Verification items for the finished model (mm, model axes). Coordinates: 2 decimals unless noted, no trailing zeros. Order: outer loops, then holes, each group sorted by start corner. A loop starts at its lowest first (then second) coordinate and runs counter-clockwise, first axis right, second up. Notation, with made-up numbers: (49.25, 26.5) -> (78.25, 26.5) arc R20 cw to (78.25, 44.5) -> close; hole circle Ø8 at (62, 29). An arc over 180 degrees is marked (long way). Write item = value, one per line. Start each with the question number.
1. Release check for a two-part mould opening along Z. For faces 1 (the cylindrical face through (0, 2, -1)), 2 (the cylindrical face through (0.108, -0.056, 0.488)), 3 (the flat face through (-1, 0, -1)) record: +Z half, -Z half, draft (parallel to the pull), parting line (faces both ways), or undercut.
2. Cross-section at A-A on x = 0. Record the cut outline in (y, z), plus the area to 3 significant figures.
3. Cross-section at B-B on y = -3. Record the cut outline in (x, z), plus the area to 3 significant figures.
4. Thickness scan on line 1 along Z through (x, y) = (0, 1); line 2 along Z through (x, y) = (-0.3, -2.75). Record the ranges inside material, lowest first. Write a range as from..to.
5. Go/stop test with flat-tipped pins: P1, Ø1, axis at y = 0, z = 1, coming from the -X side; P2, Ø1.5, axis at x = 1.5, y = -2.5, coming from the -Z side. Record where each tip stops, or that it passes through.
6. Cross-section at C-C on y = 1.25. Record the cut outline in (x, z), plus the area to 3 significant figures.
Autodesk Inventor part; units mm, degrees
ref_plane "工作平面1" through (0, -4, 0) normal (0, 1, 0) x (-1, 0, 0)
ref_plane "YZ Plane" through (0, 0, 0) normal (1, 0, 0) x (0, 1, 0)
ref_plane "XY Plane" through (0, 0, 0) normal (0, 0, 1) x (1, 0, 0)
sketch "草图1" plane through (0, 0, 0) normal (0, 1, 0) x (-1, 0, 0)
  circle A0 centre (0, 0) radius 2
  dimension "d0" = 4
ref_plane "工作平面1" through (0, -4, 0) normal (0, 1, 0) x (-1, 0, 0)
sketch "草图2" plane through (0, -4, 0) normal (0, 1, 0) x (-1, 0, 0)
  circle A0 centre (0, 0) radius 1
  dimension "d2" = 2
loft "放样1" add profiles "草图1", "草图2"
sketch "草图3" plane through (0, 0, 0) normal (0, 1, 0) x (1, 0, 0)
  circle A0 centre (0, 0) radius 1
  dimension "d7" = 2
extrude "拉伸1" add sketch "草图3" along normal blind 4
sketch "草图4" plane through (0, -4, 0) normal (0, 1, 0) x (-1, 0, 0)
  circle A0 centre (0, 0) radius 0.5
  dimension "d10" = 1
extrude "拉伸2" cut sketch "草图4" along normal through all
properties part number "conver"
Worked out:
q1.face_1 = parting line
q1.face_2 = undercut
q1.face_3 = draft
q2.outline = (-4, -1) -> (0, -2) -> (0, -1) -> (4, -1) -> (4, -0.5) -> (-4, -0.5) -> close; (-4, 0.5) -> (4, 0.5) -> (4, 1) -> (0, 1) -> (0, 2) -> (-4, 1) -> close
q2.area = 12.0 mm²
q3.outline = circle Ø2.5 at (0, 0); hole circle Ø1 at (0, 0)
q3.area = 4.12 mm²
q4.line_1 = -1..-0.5, 0.5..1
q4.line_2 = -1.28..-0.4, 0.4..1.28
q5.P1 = -1.94
q5.P2 = -1.2
q6.outline = circle Ø2 at (0, 0); hole circle Ø1 at (0, 0)
q6.area = 2.36 mm²
